Source: CAD feature listing. Evaluate the final solid. Frame: model axes, mm. A direction names the side the tool comes from. Give positions to 0.01 mm unless a question says otherwise; leave off trailing zeros. Loops run counter-clockwise (first coordinate to the right, second up) from the corner with the lowest first, then second, coordinate; pieces in that order, holes last. Notation, with made-up numbers: (36, 18) -> (83, 18) arc R7 cw to (83, 27) -> close; hole circle Ø11 at (-36.5, -2). An arc over 180 degrees is marked (long way). Put each result on its own line as item: value.
```python
from build123d import *

# Parameters (mm, degrees)
SKETCH_1_W          = 60.60764715
SKETCH_1_H          = 24.895940982
EXTRUDE_1_DEPTH     = 13.8
SKETCH_2_W          = 12.5
SKETCH_2_H          = 10.5
CUT_EXTRUDE_1_DEPTH = 42.576070048
SKETCH_3_W          = 12.5
SKETCH_3_H          = 10.5
EXTRUDE_2_DEPTH     = 0.5
SKETCH_4_R          = 2
CUT_EXTRUDE_2_DEPTH = 42.278610196
SKETCH_5_R          = 2.975
EXTRUDE_3_DEPTH     = 7.5
SKETCH_10_W         = 10.431635196
SKETCH_10_H         = 11.456709174
EXTRUDE_4_DEPTH     = 6.5
SKETCH_14_R         = 2.850486714
SKETCH_14_R_2       = 2
EXTRUDE_5_DEPTH     = 1.5
SKETCH_22_R         = 11.026465904
CUT_EXTRUDE_5_DEPTH = 42.573227563
FILLET_1_R          = 3
FILLET_2_R          = 3
FILLET_3_R          = 3
FILLET_4_R          = 3


# Read off the part's stored shape, not the designer's step: M3 螺紋孔3
with BuildPart() as part:
    # 草圖1 → 填料-伸長1 (new body)
    with BuildSketch(Plane(origin=(0, 0, 0), x_dir=(1, 0, 0), z_dir=(0, 1, 0))):
        Rectangle(SKETCH_1_W, SKETCH_1_H)
    extrude(amount=EXTRUDE_1_DEPTH)

    # 草圖2 → 除料-伸長1 (cut, through all)
    with BuildSketch(Plane.XY.offset(12.447970491)):
        with Locations((18, 7.5)):
            Rectangle(SKETCH_2_W, SKETCH_2_H)
    extrude(amount=-CUT_EXTRUDE_1_DEPTH, mode=Mode.SUBTRACT)

    # 草圖3 → 填料-伸長2 (add)
    with BuildSketch(Plane.XY.offset(12.447970491)):
        with Locations((18, 7.5)):
            Rectangle(SKETCH_3_W, SKETCH_3_H)
    extrude(amount=-EXTRUDE_2_DEPTH)

    # 草圖4 → 除料-伸長2 (cut, through all)
    with BuildSketch(Plane(origin=(0, 0, 11.947970491), x_dir=(-1, 0, 0), z_dir=(0, 0, -1))):
        with Locations((-18, 7.5)):
            Circle(SKETCH_4_R)
    extrude(amount=-CUT_EXTRUDE_2_DEPTH, mode=Mode.SUBTRACT)

    # 草圖5 → 填料-伸長3 (add)
    with BuildSketch(Plane.XY.offset(12.447970491)):
        with Locations(Location((-15.151911787, 6.9, 0), (0, 0, 180))):
            Circle(SKETCH_5_R)
    extrude(amount=EXTRUDE_3_DEPTH)

    # 草圖10 → 填料-伸長4 (add)
    with BuildSketch(Plane(origin=(0, 13.8, 0), x_dir=(1, 0, 0), z_dir=(0, 1, 0))):
        with Locations((0, 4.510890299)):
            Rectangle(SKETCH_10_W, SKETCH_10_H)
    extrude(amount=EXTRUDE_4_DEPTH)

    # M3 螺紋孔3 outline → M3 螺紋孔3 (revolve, cut)
    with BuildSketch(Plane.XY.offset(-8.13268367)):
        Polygon((0, 0), (1.25, 0), (1.25, 20.069247601), (1.525, 20.3), (0, 20.3), align=None)
    revolve(axis=Axis((0, 0, -8.13268367), (0, 1, 0)), mode=Mode.SUBTRACT)

    # Hole Wizard M3 _3 2 outline → Hole Wizard M3 _3 2 (revolve, cut)
    with BuildSketch(Plane.XY.offset(-0.83268367)):
        Polygon((0, 0), (1.25, 0), (1.25, 20.069247601), (1.525, 20.3), (0, 20.3), align=None)
    revolve(axis=Axis((0, 0, -0.83268367), (0, 1, 0)), mode=Mode.SUBTRACT)

    # 草圖14 → 填料-伸長5 (add)
    with BuildSketch(Plane.XY.offset(12.447970491)):
        with Locations(Location((18, 7.5, 0), (0, 0, 180))):
            Circle(SKETCH_14_R)
        with Locations(Location((18, 7.5, 0), (0, 0, 180))):
            Circle(SKETCH_14_R_2, mode=Mode.SUBTRACT)
    extrude(amount=EXTRUDE_5_DEPTH)

    # 草圖22 → 除料-伸長5 (cut, through all)
    with BuildSketch(Plane.XZ):
        with Locations(Location((-16.460754219, 0, 0), (0, 0, 270))):
            Circle(SKETCH_22_R)
    extrude(amount=-CUT_EXTRUDE_5_DEPTH, mode=Mode.SUBTRACT)

    # 圓角1
    fillet_1_edges = [part.edges().sort_by_distance(p)[0] for p in [
        (-30.303823575, 6.9, -12.447970491),
    ]]
    fillet(fillet_1_edges, radius=FILLET_1_R)

    # 圓角2
    fillet_2_edges = [part.edges().sort_by_distance(p)[0] for p in [
        (-30.303823575, 6.9, 12.447970491),
    ]]
    fillet(fillet_2_edges, radius=FILLET_2_R)

    # 圓角3
    fillet_3_edges = [part.edges().sort_by_distance(p)[0] for p in [
        (30.303823575, 6.9, -12.447970491),
    ]]
    fillet(fillet_3_edges, radius=FILLET_3_R)

    # 圓角4
    fillet_4_edges = [part.edges().sort_by_distance(p)[0] for p in [
        (30.303823575, 6.9, 12.447970491),
    ]]
    fillet(fillet_4_edges, radius=FILLET_4_R)


solid = part.part
```
(1) Section B-B on y = 6.9. Return loops of the section in (x, z), then the cut area to 3 significant figures.
Calculated:
outline: (-30.3, -9.45) arc R3 ccw to (-27.3, -12.45) -> (11.75, -12.45) -> (11.75, 11.95) -> (16.09, 11.95) -> (16.09, 13.95) -> (15.21, 13.95) -> (15.21, 12.45) -> (-12.18, 12.45) -> (-12.18, 19.95) -> (-18.13, 19.95) -> (-18.13, 12.45) -> (-27.3, 12.45) arc R3 ccw to (-30.3, 9.45) -> close; (19.91, 11.95) -> (24.25, 11.95) -> (24.25, -12.45) -> (27.3, -12.45) arc R3 ccw to (30.3, -9.45) -> (30.3, 9.45) arc R3 ccw to (27.3, 12.45) -> (20.79, 12.45) -> (20.79, 13.95) -> (19.91, 13.95) -> close; hole circle Ø22.05 at (-16.46, 0); hole circle Ø2.5 at (0, -8.13); hole circle Ø2.5 at (0, -0.83)
area: 850 mm²
(2) Section C-C on z = 4.5. Return loops of the section in (x, y).
Calculated:
outline: (-30.3, 0) -> (-26.53, 0) -> (-26.53, 13.8) -> (-30.3, 13.8) -> close; (-6.39, 0) -> (30.3, 0) -> (30.3, 13.8) -> (-6.39, 13.8) -> close; hole (11.75, 2.25) -> (24.25, 2.25) -> (24.25, 12.75) -> (11.75, 12.75) -> close
(3) Draft query along Y for faces 1 (the flat face through (18, 2.25, 0)), 2 (the cylindrical face through (-12.79, 8.71, 16.15)), 3 (the flat face through (0, 7, 12.448)). Return one class per face: released by +Y, released by -Y, zero draft, split by the parting line, or undercut.
Calculated:
face 1: undercut
face 2: split by the parting line
face 3: zero draft
(4) Section D-D on x = 18. Return loops of the section in (y, z).
Calculated:
outline: (0, -12.45) -> (2.25, -12.45) -> (2.25, 11.95) -> (5.5, 11.95) -> (5.5, 13.95) -> (4.65, 13.95) -> (4.65, 12.45) -> (0, 12.45) -> close; (9.5, 11.95) -> (12.75, 11.95) -> (12.75, -12.45) -> (13.8, -12.45) -> (13.8, 12.45) -> (10.35, 12.45) -> (10.35, 13.95) -> (9.5, 13.95) -> close
(5) Section A-A on x = 0. Return loops of the section in (y, z), then the cut area to 3 significant figures.
Calculated:
outline: (0, -12.45) -> (13.8, -12.45) -> (13.8, -10.24) -> (20.3, -10.24) -> (20.3, -9.66) -> (20.07, -9.38) -> (0, -9.38) -> close; (0, -6.88) -> (20.07, -6.88) -> (20.3, -6.61) -> (20.3, -2.36) -> (20.07, -2.08) -> (0, -2.08) -> close; (0, 0.42) -> (20.07, 0.42) -> (20.3, 0.69) -> (20.3, 1.22) -> (13.8, 1.22) -> (13.8, 12.45) -> (0, 12.45) -> close
area: 316 mm²
(6) Line query: probe 1 along Z at (x, y) = (0, 6); probe 2 along Y at (x, z) = (23, 0.5); probe 3 along X at (y, z) = (9, 6). Output: solid intervals per line, ascending. Write a range as from..to.
Calculated:
probe 1: z = -12.45..-9.38, -6.88..-2.08, 0.42..12.45
probe 2: y = 0..2.25, 12.75..13.8
probe 3: x = -30.3..-25.71, -7.21..11.75, 24.25..30.3
(7) First-contact query: P1, Ø7, axis at x = 0.5, y = 18, coming from the +Z side; P2, Ø10, axis at x = 20, y = 10, coming from the -Z side; P3, Ø2, axis at y = 17.5, z = -7, coming from the +X side; P4, Ø2, axis at x = 0, z = -0.83, coming from the -Y side. Flat tips, straight axial feed; report the tip coordinate or a pass-through.
Calculated:
P1: stops at z = 1.22
P2: stops at z = -12.45
P3: stops at x = 5.22
P4: passes through
(8) Reachability of faces 4 (the flat face through (0, 17, 1.217)), 5 (the flat face through (-5.216, 17, -4)), 6 (the flat face through (11.75, 7, 0)), 7 (the cylindrical face through (20.262, 9.234, 13.187)), 8 (the cylindrical face through (29.448, 6.997, 11.546)) from +Z, -Z, +X, -X, +Y, -Y: full face, straight path, thin tool, end or side. Return the list, or none.
Calculated:
face 4: +Z, +X, -X, +Y
face 5: +Z, -Z, -X, +Y
face 6: -Z
face 7: +Z
face 8: +Z, +X, +Y, -Y
